from build123d import *

# Parameters (mm, degrees)
SKETCH_2_W                 = 210.5009
SKETCH_2_H                 = 77.1505
EXTRUDE_1_DEPTH            = 34.5
SHELL_1_T                  = -10
SHELL_1_THICKNESS_2_FACE_W = 190.5009
SHELL_1_THICKNESS_2_FACE_H = 57.1505
SHELL_1_THICKNESS_2_DEPTH  = 7
SKETCH_3_R                 = 2.1
CUT_EXTRUDE_8_DEPTH        = 7.6
SKETCH_4_R                 = 5
EXTRUDE_2_DEPTH            = 9.1
SKETCH_6_R                 = 1.55
CUT_EXTRUDE_9_DEPTH        = 9.1
CUT_EXTRUDE_START          = 12.1
SKETCH_10_OUTSIDE_W        = 257.867
SKETCH_10_OUTSIDE_H        = 124.516
SKETCH_10_OUTSIDE_R        = 3
CUT_EXTRUDE_16_DEPTH       = 4.6
FILLET_1_R                 = 2


with BuildPart() as part:
    # 草图2 → 凸台-拉伸1 (new body)
    with BuildSketch(Plane.XY):
        with Locations((95.3455423, 28.832065)):
            Rectangle(SKETCH_2_W, SKETCH_2_H)
    extrude(amount=EXTRUDE_1_DEPTH)

    # 抽壳1
    shell_1_openings = [part.faces().sort_by_distance(p)[0] for p in [
        (95.3455423, 28.832065, 34.5),
    ]]
    offset(amount=SHELL_1_T, openings=shell_1_openings, kind=Kind.INTERSECTION)

    # 抽壳1 thickness 2 face (on inner face of the shell) → 抽壳1 thickness 2 (cut)
    with BuildSketch(Plane(origin=(95.3455423, 28.832065, 10), x_dir=(-1, 0, 0), z_dir=(0, 0, -1))):
        Rectangle(SHELL_1_THICKNESS_2_FACE_W, SHELL_1_THICKNESS_2_FACE_H)
    extrude(amount=SHELL_1_THICKNESS_2_DEPTH, mode=Mode.SUBTRACT)

    # 草图3 → 切除-拉伸8 (cut)
    with BuildSketch(Plane.XY):
        with Locations(Location((38.19575, 38.357, 0), (0, 0, 180))):
            Circle(SKETCH_3_R)
    extrude(amount=CUT_EXTRUDE_8_DEPTH, mode=Mode.SUBTRACT)

    # 草图4 → 凸台-拉伸2 (add)
    with BuildSketch(Plane.XY.offset(3)):
        with Locations((38.19575, 38.357)):
            Circle(SKETCH_4_R)
    extrude(amount=EXTRUDE_2_DEPTH)

    # 草图6 → 切除-拉伸9 (cut)
    with BuildSketch(Plane.XY.offset(12.1)):
        with Locations((38.19575, 38.357)):
            Circle(SKETCH_6_R)
    extrude(amount=-CUT_EXTRUDE_9_DEPTH, mode=Mode.SUBTRACT)

    # 草图10 outside → 切除-拉伸16 (cut)
    with BuildSketch(Plane.XY.offset(CUT_EXTRUDE_START)):
        with Locations((95.3455, 28.832)):
            Rectangle(SKETCH_10_OUTSIDE_W, SKETCH_10_OUTSIDE_H)
        with Locations((38.19575, 38.357)):
            Circle(SKETCH_10_OUTSIDE_R, mode=Mode.SUBTRACT)
    extrude(amount=-CUT_EXTRUDE_16_DEPTH, mode=Mode.SUBTRACT)


with BuildPart() as cut_extrude_16_kept_piece:
    # of the separate pieces the step leaves, the one the design keeps (cut_extrude_16_pieces_kept)
    add(part.part.solids().sort_by_distance((200.5959923, -9.743185, 0))[0])

    # 圆角1
    fillet_1_edges = [cut_extrude_16_kept_piece.edges().sort_by_distance(p)[0] for p in [
        (-9.9049077, 28.832065, 7.5),
        (95.3455423, -9.743185, 7.5),
        (200.5959923, 28.832065, 7.5),
        (95.3455423, 67.407315, 7.5),
    ]]
    fillet(fillet_1_edges, radius=FILLET_1_R)


solid = cut_extrude_16_kept_piece.part
Verification items for the finished model (mm, model axes). A direction names the side the tool comes from. Coordinates: 2 decimals unless noted, no trailing zeros. Order: outer loops, then holes, each group sorted by start corner. A loop starts at its lowest first (then second) coordinate and runs counter-clockwise, first axis right, second up. Notation, with made-up numbers: (69, 18) -> (76, 18) arc R18 cw to (76, 36) -> close; hole circle Ø4 at (38, 76). An arc over 180 degrees is marked (long way). Put each result on its own line as item: value. Start each with the question number.
1. Access from +Z, -Z, +X, -X, +Y, -Y to the whole of each face (thin tool, end or side, straight path). Record for faces 1 (the flat face through (37, 37, 3)), 2 (the flat face through (-9.905, 28, 3)), 3 (the flat face through (0.095, 28, 5)).
2. Go/stop test with flat-tipped pins: pin 1 Ø2 at (x, y) = (120, 29) entering from +Z; pin 2 Ø4 at (x, y) = (37, 43.5) entering from +Z; pin 3 Ø3.5 at (x, y) = (38, 39.5) entering from -Z; pin 4 Ø4 at (x, y) = (38.2, 38.36) entering from -Z. Record where each tip stops, or that it passes through.
3. Cross-section at A-A, the plane y = 18. Record the boundary of the cut face in (x, z), then the cut area to 3 significant figures.
4. Mould release check, pull along Y, two halves, no side actions. Record for faces 4 (the flat face through (94, -9.743, 3)), 5 (the cylindrical face through (36.256, 39.161, 1.479)), 6 (the cylindrical face through (35.2, 38.5, 9.8)): released by +Y, released by -Y, zero draft, split by the parting line, or undercut.
5. Cross-section at B-B, the plane x = 137. Record the boundary of the cut face in (y, z), then the cut area to 3 significant figures.
6. Material ranges on L1, parallel to Y at x = 139.5, z = 3.5; L2, parallel to Z at x = 17, y = 5; L3, parallel to Z at x = 139, y = 60.5, recorded low to high. Write a range as [from, to].
Computed:
1. face 1: -Z
1. face 2: +Z, -Z, -X, +Y, -Y
1. face 3: +Z
2. pin 1: z = 3
2. pin 2: z = 7.5
2. pin 3: z = 0
2. pin 4: z = 3
3. outline: (-9.9, 0) -> (200.6, 0) -> (200.6, 5.5) arc R2 ccw to (198.6, 7.5) -> (190.6, 7.5) -> (190.6, 3) -> (0.1, 3) -> (0.1, 7.5) -> (-7.9, 7.5) arc R2 ccw to (-9.9, 5.5) -> close
3. area: 720 mm2
4. face 4: released by -Y
4. face 5: undercut
4. face 6: split by the parting line
5. outline: (-9.74, 0) -> (67.41, 0) -> (67.41, 5.5) arc R2 ccw to (65.41, 7.5) -> (57.41, 7.5) -> (57.41, 3) -> (0.26, 3) -> (0.26, 7.5) -> (-7.74, 7.5) arc R2 ccw to (-9.74, 5.5) -> close
5. area: 320 mm2
6. L1: [-9.74, 0.26], [57.41, 67.41]
6. L2: [0, 3]
6. L3: [0, 7.5]
